from build123d import *

# Parameters (mm, degrees)
F0_W     = 76.2
F0_H     = 76.2
F1_DEPTH = 25.4
F2_SIZE2 = 25.39999
F2_SIZE  = 25.39999
F3_SIZE2 = 17.785261
F3_SIZE  = 25.39999
F4_SIZE2 = 25.39999
F4_SIZE  = 25.39999
F5_SIZE2 = 25.39999
F5_SIZE  = 25.39999


# Not quite as in the source:
# - a fillet or chamfer is up to 0.001 mm smaller than in the source, because OpenCascade refuses the exact size


with BuildPart() as f1:
    # F0 (on Top) → F1 (new body)
    with BuildSketch(Plane.XY):
        with Locations((-5.1121336523, -3.4328531474)):
            Rectangle(F0_W, F0_H)
    extrude(amount=F1_DEPTH)

    # F2 (size 25.4 and 25.4 in the source; OpenCascade refuses exactly that, so slightly less here)
    f2_edges = [f1.edges().sort_by_distance(p)[0] for p in [
        (32.987866, -3.432853, 25.4),
    ]]
    chamfer(f2_edges, length=F2_SIZE, length2=F2_SIZE2)

    # F3 (size 25.4 and 17.7852714705 in the source; OpenCascade refuses exactly that, so slightly less here)
    f3_edges = [f1.edges().sort_by_distance(p)[0] for p in [
        (-17.812129, 34.667147, 25.4),
    ]]
    f3_side = f1.faces().sort_by_distance((-11.038795, 34.667147, 11.853333))[0]
    chamfer(f3_edges, length=F3_SIZE, length2=F3_SIZE2, reference=f3_side)

    # F4 (size 25.4 and 25.4 in the source; OpenCascade refuses exactly that, so slightly less here)
    f4_edges = [f1.edges().sort_by_distance(p)[0] for p in [
        (-43.212134, -12.325484, 25.4),
    ]]
    chamfer(f4_edges, length=F4_SIZE, length2=F4_SIZE2)

    # F5 (size 25.4 and 25.4 in the source; OpenCascade refuses exactly that, so slightly less here)
    f5_edges = [f1.edges().sort_by_distance(p)[0] for p in [
        (-5.112134, -41.532853, 25.4),
    ]]
    chamfer(f5_edges, length=F5_SIZE, length2=F5_SIZE2)


solid = f1.part
Could you check a few things on this model? Use its own coordinates, in mm. Give positions to 0.01 mm unless a question says otherwise; leave off trailing zeros. Order: outer loops, then holes, each group sorted by start corner. A loop starts at its lowest first (then second) coordinate and runs counter-clockwise, first axis right, second up.
1. Will these pins go through, and if not, where does the flat tip stop? P1, Ø10, axis at y = -5.5, z = 14.5, coming from the -X side; P2, Ø3, axis at y = -11, z = 10, coming from the +X side; P3, Ø1, axis at x = 11, z = 3, coming from the +Y side.
2. I need wall thicknesses on L1, parallel to Y at x = -11, z = 13.25; L2, parallel to X at y = -22.5, z = 1.5; L3, parallel to Z at x = 21, y = -11. Which ranges of each line are inside material? Lowest first, please.
3. Suppose I cut it at D-D (z = 17). List the corners of the cut face in (x, y) for me.
4. We'd pull the mould along Z, two halves only. Please class faces 1 (the flat face through (-5.646, 27.626, 10.056)), 2 (the flat face through (-6, -3, 0)): pulls with the +Z half, pulls with the -Z half, needs draft (parallel to the pull), parting line crosses it, or undercut.
5. Suppose I cut it at C-C (z = 21.5). List the corners of the cut face in (x, y) for me.
Solved:
1. P1: stops at x = -33.71
1. P2: stops at x = 24.49
1. P3: stops at y = 32.92
2. L1: y = -28.28 to 25.39
2. L2: x = -41.71 to 31.49
2. L3: z = 0 to 11.99
3. outline: (-26.21, -24.53) - (15.99, -24.53) - (15.99, 22.76) - (-26.21, 22.76) - close
4. face 1: pulls with the +Z half
4. face 2: pulls with the -Z half
5. outline: (-21.71, -20.03) - (11.49, -20.03) - (11.49, 19.61) - (-21.71, 19.61) - close
